The listing builds one solid part. Answer for the finished solid, in the listing's coordinates (mm). Face numbers are marked on the shaded views. A direction names the side the tool comes from. Coordinates: 2 decimals unless noted, no trailing zeros. Loops run counter-clockwise (first coordinate to the right, second up) from the corner with the lowest first, then second, coordinate; pieces in that order, holes last. Notation, with made-up numbers: (-1.75, 88) - (22.25, 88) arc R11 ccw to (22.25, 92) - close; hole circle Ø11 at (18.5, 17.5). An arc over 180 degrees is marked (long way). Return JSON: item names as keys, results as strings. Group by question number.
1. Section B-B (y = 24.5) is taken. Write down the section's boundary in (x, z), and give its area (3 significant figures).
2. The mould has two halves that part along Z. Classify the marked faces 1, 2, 3 and 4: pulls with the +Z half, pulls with the -Z half, needs draft (parallel to the pull), parting line crosses it, or undercut.
3. Find the intervals of material crossed by line 1 along Y through (x, z) = (9.8, 0); line 2 along Z through (x, y) = (0, 12.5); line 3 along Z through (x, y) = (8.6, 24.5), in increasing order.
4. Each of these flat-tipped pins is pushed along its axis until it touches: P1, Ø1.5, axis at x = -8, y = 19.5, coming from the -Z side; P2, Ø1.7, axis at y = 24.5, z = 8, coming from the +X side; P3, Ø11, axis at x = -4.5, y = 21.5, coming from the -Z side. Where does it stop, or does it pass through?
5. Section D-D (x = 4) is taken. Write down the section's boundary in (y, z), and give its area (3 significant figures).
6. Section C-C (y = 12.25) is taken. Write down the section's boundary in (x, z), and give its area (3 significant figures).
7. Which of the six approach directions +Z, -Z, +X, -X, +Y, -Y give full straight-line access (tool end or side, diameter ignored) to the marked faces 5, 6, 7 and 8?
8. Section A-A (x = 0) is taken. Write down the section's boundary in (y, z).
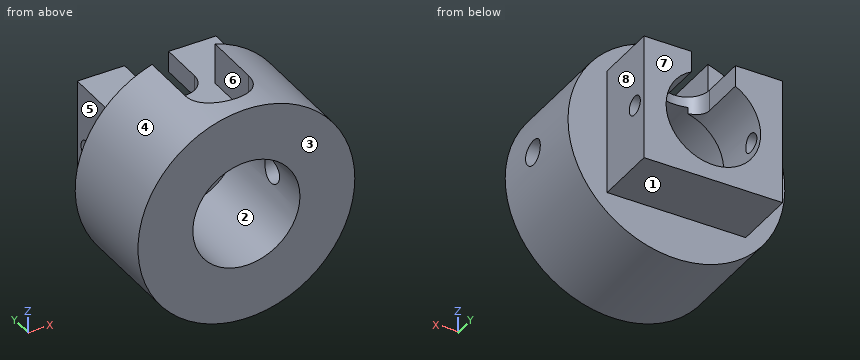
```python
from build123d import *

# Parameters (mm, degrees)
SKETCH1_R           = 17.2
SKETCH1_R_2         = 8.5
BOSS_EXTRUDE1_DEPTH = 17
SKETCH2_W           = 22
SKETCH2_H           = 20
SKETCH2_R           = 7.5
BOSS_EXTRUDE2_DEPTH = 10
SKETCH3_R           = 1.5
CUT_EXTRUDE1_DEPTH  = 22
SKETCH4_R           = 2
CUT_EXTRUDE2_DEPTH  = 20
CUT_EXTRUDE3_DEPTH  = 20
CUT_EXTRUDE4_DEPTH  = 5


with BuildPart() as part:
    # Sketch1 → Boss-Extrude1 (new body)
    with BuildSketch(Plane(origin=(0, 0, 0), x_dir=(1, 0, 0), z_dir=(0, 1, 0))):
        Circle(SKETCH1_R)
        Circle(SKETCH1_R_2, mode=Mode.SUBTRACT)
    extrude(amount=BOSS_EXTRUDE1_DEPTH)

    # Sketch2 → Boss-Extrude2 (add)
    with BuildSketch(Plane(origin=(0, 17, 0), x_dir=(1, 0, 0), z_dir=(0, 1, 0))):
        Rectangle(SKETCH2_W, SKETCH2_H)
        Circle(SKETCH2_R, mode=Mode.SUBTRACT)
    extrude(amount=BOSS_EXTRUDE2_DEPTH)

    # Sketch3 → Cut-Extrude1 (cut)
    with BuildSketch(Plane(origin=(11, 0, 0), x_dir=(0, 0, -1), z_dir=(1, 0, 0))):
        with Locations((0, 24.5)):
            Circle(SKETCH3_R)
    extrude(amount=-CUT_EXTRUDE1_DEPTH, mode=Mode.SUBTRACT)

    # Sketch4 → Cut-Extrude2 (cut)
    with BuildSketch(Plane(origin=(0, 0, 0), x_dir=(0, 0, -1), z_dir=(1, 0, 0))):
        with Locations((0, 7.5)):
            Circle(SKETCH4_R)
    extrude(amount=CUT_EXTRUDE2_DEPTH, mode=Mode.SUBTRACT)

    # Sketch5 → Cut-Extrude3 (cut)
    with BuildSketch(Plane.XY.offset(10)):
        with BuildLine():
            Line((-5, 17), (5, 17))
            Line((5, 17), (5, 8))
            ThreePointArc((5, 8), (0, 3), (-5, 8))
            Line((-5, 8), (-5, 17))
        make_face()
    extrude(amount=CUT_EXTRUDE3_DEPTH, mode=Mode.SUBTRACT)

    # Sketch6 → Cut-Extrude4 (cut)
    with BuildSketch(Plane.XY.offset(10)):
        with BuildLine():
            Line((3.5, 27), (-3.5, 27))
            Line((-3.5, 27), (-3.5, 20))
            ThreePointArc((-3.5, 20), (0, 16.5), (3.5, 20))
            Line((3.5, 20), (3.5, 27))
        make_face()
    extrude(amount=-CUT_EXTRUDE4_DEPTH, mode=Mode.SUBTRACT)


solid = part.part
```
The answers:
{
 "1": {"outline": "(-11, -10) - (11, -10) - (11, -1.5) - (7.35, -1.5) arc R7.5 cw to (-7.35, -1.5) - (-11, -1.5) - close; (-11, 1.5) - (-7.35, 1.5) arc R7.5 cw to (-3.5, 6.63) - (-3.5, 10) - (-11, 10) - close; (3.5, 6.63) arc R7.5 cw to (7.35, 1.5) - (11, 1.5) - (11, 10) - (3.5, 10) - close", "area": "223 mm2"},
 "2": {"face 1": "pulls with the -Z half", "face 2": "undercut", "face 3": "needs draft", "face 4": "parting line crosses it"},
 "3": {"line 1": "y = 0 to 5.5, 9.5 to 23, 26 to 27", "line 2": "z = -17.2 to -8.5, 8.5 to 10", "line 3": "z = -10 to -1.5, 1.5 to 10"},
 "4": {"P1": "stops at z = -10", "P2": "stops at x = 11", "P3": "stops at z = -17.15"},
 "5": {"outline": "(0, -16.73) - (17, -16.73) - (17, -10) - (27, -10) - (27, -6.34) - (17, -6.34) - (17, -7.5) - (0, -7.5) - close; (0, 7.5) - (17, 7.5) - (17, 6.34) - (27, 6.34) - (27, 10) - (5, 10) - (5, 16.73) - (0, 16.73) - close", "area": "306 mm2"},
 "6": {"outline": "(-5, 10) - (-5, 16.46) arc R17.2 ccw (long way) to (5, 16.46) - (5, 10) - close; hole circle Ø17 at (0, 0)", "area": "633 mm2"},
 "7": {"face 5": "+Z, -Z, -X, +Y", "face 6": "+Z, +Y", "face 7": "+Z, -Z, +X, -X, +Y", "face 8": "+Z, -Z, +X, +Y"},
 "8": {"outline": "(0, -17.2) - (17, -17.2) - (17, -10) - (27, -10) - (27, -7.5) - (17, -7.5) - (17, -8.5) - (0, -8.5) - close; (0, 8.5) - (16.5, 8.5) - (16.5, 10) - (3, 10) - (3, 17.2) - (0, 17.2) - close"}
}
